Work out the finished part from the listing and answer in its coordinate system (mm). A direction names the side the tool comes from. Give positions to 0.01 mm unless a question says otherwise; leave off trailing zeros. Order: outer loops, then holes, each group sorted by start corner. A loop starts at its lowest first (then second) coordinate and runs counter-clockwise, first axis right, second up. Notation, with made-up numbers: (20, 0.25) -> (32, 0.25) arc R6 cw to (32, 6.25) -> close; hole circle Ø2 at (-17, -21). An arc over 180 degrees is marked (long way). Use a Markdown table: item, result. Add a question column.
Autodesk Inventor part; units mm, degrees
ref_plane "YZ Plane" through (0, 0, 0) normal (1, 0, 0) x (0, 1, 0)
ref_plane "XZ Plane" through (0, 0, 0) normal (0, 1, 0) x (-1, 0, 0)
ref_plane "XY Plane" through (0, 0, 0) normal (0, 0, 1) x (1, 0, 0)
sketch "Sketch1" plane through (0, 0, 0) normal (0, 1, 0) x (-1, 0, 0)
  line L0 (0, 0) -> (304.8083, 0)
  line L1 (304.8083, 0) -> (304.8083, -25.4)
  line L2 (304.8083, -25.4) -> (0, -25.4)
  line L3 (0, -25.4) -> (0, 0)
  dimension "d0" = 25.4
extrude "Extrusion1" add sketch "Sketch1" along normal blind 6.35
fillet "Fillet1" radius 12.7 1 edges at (-304.8083, 3.175, -25.4)
fillet "Fillet2" radius 12.7 1 edges at (-304.8083, 3.175, 0)
fillet "Fillet3" radius 12.7 1 edges at (0, 3.175, 0)
fillet "Fillet4" radius 12.7 1 edges at (0, 3.175, -25.4)
shell "Shell1" thickness 2.54 removed faces 2 at (-198.9723, 6.35, -8.4667) at (-198.9723, 0, -8.4667)
properties part number "LiftLineWire"
1) The part is cut by section A-A, the plane x = -157. Determine the outline of the cut face in (y, z), then the cut area to 3 significant figures.
2) Flat-ended cylindrical pins translate along their axes: pin 1 (2 mm diameter, centred on x = -230, z = -20.5, fed in from -Y); pin 2 (2 mm diameter, centred on y = 2.5, z = -3.5, fed in from -X); pin 3 (2 mm diameter, centred on y = 3, z = -11, fed in from -X). Find the tip coordinate at first contact, or state that the pin passes through.
3) Which of the six approach directions +Z, -Z, +X, -X, +Y, -Y give full straight-line access (tool end or side, diameter ignored) to faces 4 (the cylindrical face through (-299.213, 3.219, -19.963)), 5 (the cylindrical face through (-3.62, 3.22, -21.58))?
4) The part is cut by section C-C, the plane z = -8. Determine the outline of the cut face in (x, y).
5) Straight lines are drawn through the part: line 1 (Z direction, x = -30, y = 1.75); line 2 (X direction, y = 5.5, z = -4.25); line 3 (X direction, y = 3.5, z = -8). For each, find the intervals that lie inside material, in ascending order.
6) Determine the mould class of faces 1 (the cylindrical face through (-5.437, 3.219, -19.805)), 2 (the cylindrical face through (-301.19, 3.22, -3.82)), 3 (the cylindrical face through (-300.99, 3.22, -21.78)) for opening direction Z: released by +Z, released by -Z, zero draft, split by the parting line, or undercut.
A:
| question | item | result |
|---|---|---|
| 1 | outline | (0, -25.4) -> (6.35, -25.4) -> (6.35, -22.86) -> (0, -22.86) -> close; (0, -2.54) -> (6.35, -2.54) -> (6.35, 0) -> (0, 0) -> close |
| 1 | area | 32.3 mm^2 |
| 2 | pin 1 | through |
| 2 | pin 2 | x = -301.81 |
| 2 | pin 3 | x = -304.79 |
| 3 | face 4 | +Y, -Y |
| 3 | face 5 | -Z, +X, +Y, -Y |
| 4 | outline | (-303.91, 0) -> (-301.12, 0) -> (-301.12, 6.35) -> (-303.91, 6.35) -> close; (-3.69, 0) -> (-0.9, 0) -> (-0.9, 6.35) -> (-3.69, 6.35) -> close |
| 5 | line 1 | -25.4 to -22.86, -2.54 to 0 |
| 5 | line 2 | -301.59 to -297.75, -7.06 to -3.22 |
| 5 | line 3 | -303.91 to -301.12, -3.69 to -0.9 |
| 6 | face 1 | undercut |
| 6 | face 2 | released by +Z |
| 6 | face 3 | released by -Z |
